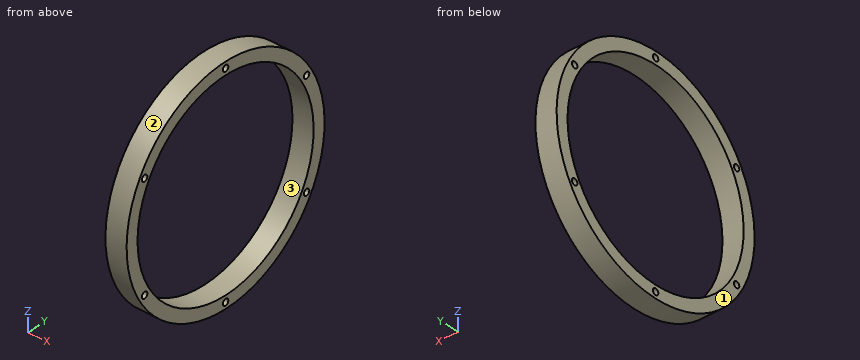
Autodesk Inventor part; units mm, degrees
ref_plane "YZ Plane" through (0, 0, 0) normal (1, 0, 0) x (0, 1, 0)
ref_plane "XZ Plane" through (0, 0, 0) normal (0, 1, 0) x (-1, 0, 0)
ref_plane "XY Plane" through (0, 0, 0) normal (0, 0, 1) x (1, 0, 0)
sketch "Sketch1" plane through (0, 0, 0) normal (0, 1, 0) x (-1, 0, 0)
  line L0 (0, -83.3) -> (0, -70.7) construction
  line L1 (-10.78, 0) -> (10.78, 0) construction
  line L2 (-7.7, -72.5) -> (7.7, -72.5)
  line L3 (-7.7, -72.5) -> (-7.7, -81.5)
  line L4 (-7.7, -81.5) -> (7.7, -81.5)
  line L5 (7.7, -81.5) -> (7.7, -72.5)
  dimension "d30" = 15.4
  dimension "d31" = 9
  dimension "d47" = 72.5
revolve "Revolution1" add sketch "Sketch1" angle 360 about axis through (0, 0, 0) along (-1, 0, 0)
sketch "Sketch2" plane through (-7.7, 0, 0) normal (-1, 0, 0) x (0, 0, 1)
  line L0 (0, 114.1) -> (0, -114.1) construction
  line L1 (-114.1, 0) -> (114.1, 0) construction
  circle A0 centre (0, 0) radius 72.5
  circle A1 centre (0, 0) radius 81.5
  circle A2 centre (0, 0) radius 77 construction
  point P0 (-77, 0)
  dimension "d33" = 4.5
  dimension "d34" = 4.5
hole "Hole1" at (-7.7, 0, -77) direction (1, 0, 0) diameter 4.5 end through all
pattern_circular "Circular Pattern1" count 6 over 360 about axis through (-10, 0, 0) along (1, 0, 0) of "Hole1"
equation "\"d33\" = d34"
equation "\"D_ring\" = D_ext"
properties part number "Adapter_stages_planetary" material "Aluminum 6061"
Input: part model. Units: mm. Frame: model coordinates. Face numbers are marked on the shaded views. Give positions to 0.01 mm unless a question says otherwise; leave off trailing zeros. Order: outer loops, then holes, each group sorted by start corner. A loop starts at its lowest first (then second) coordinate and runs counter-clockwise, first axis right, second up. Notation, with made-up numbers: (-37, 80) -> (-22, 80) arc R22 cw to (-22, 87) -> close; hole circle Ø4 at (-8, -27). An arc over 180 degrees is marked (long way). Use one line per item in the form item = value.
1) Line query: probe 1 along Z at (x, y) = (-6, 67); probe 2 along Z at (x, y) = (3.25, 37.5); probe 3 along Z at (x, y) = (4.5, -18). Output: solid intervals per line, ascending.
Response values:
probe_1 = -46.4 to -40.73, -36.27 to -27.7, 27.7 to 36.27, 40.73 to 46.4
probe_2 = -72.36 to -62.05, 62.05 to 72.36
probe_3 = -79.49 to -70.23, 70.23 to 79.49
2) Section D-D, the plane x = -1.75. Return loops of the section in (y, z) (3 decimals), and give its area (3 significant figures).
Response values:
outline = circle Ø163 at (0, 0); hole circle Ø145 at (0, 0); hole circle Ø4.5 at (-66.684, -38.5); hole circle Ø4.5 at (-66.684, 38.5); hole circle Ø4.5 at (0, -77); hole circle Ø4.5 at (0, 77); hole circle Ø4.5 at (66.684, -38.5); hole circle Ø4.5 at (66.684, 38.5)
area = 4,260 mm^2
3) First-contact query: pin 1 Ø6 at (x, z) = (3.5, 62) entering from -Y (3 decimals); pin 2 Ø4 at (x, y) = (3, -4) entering from +Z; pin 3 Ø6 at (x, z) = (-1.5, 42.5) entering from -Y. Flat tips, straight axial feed; report the tip coordinate or a pass-through.
Response values:
pin_1 = -56.225
pin_2 = 81.48
pin_3 = -71.29
4) Section A-A, the plane y = 0. Return loops of the section in (x, z).
Response values:
outline = (-7.7, -81.5) -> (7.7, -81.5) -> (7.7, -79.25) -> (-7.7, -79.25) -> close; (-7.7, -74.75) -> (7.7, -74.75) -> (7.7, -72.5) -> (-7.7, -72.5) -> close; (-7.7, 72.5) -> (7.7, 72.5) -> (7.7, 74.75) -> (-7.7, 74.75) -> close; (-7.7, 79.25) -> (7.7, 79.25) -> (7.7, 81.5) -> (-7.7, 81.5) -> close
5) Section C-C, the plane y = -22.5. Return loops of the section in (x, z).
Response values:
outline = (-7.7, -78.33) -> (7.7, -78.33) -> (7.7, -68.92) -> (-7.7, -68.92) -> close; (-7.7, 68.92) -> (7.7, 68.92) -> (7.7, 78.33) -> (-7.7, 78.33) -> close
6) Mould query, pull axis Z, two halves, no side actions, for the marked faces 1, 2 and 3. Classes: pulls with the +Z half, pulls with the -Z half, needs draft (parallel to the pull), parting line crosses it, or undercut.
Response values:
face_1 = needs draft
face_2 = parting line crosses it
face_3 = undercut
7) Section B-B, the plane z = 0. Return loops of the section in (x, y), and give its area (3 significant figures).
Response values:
outline = (-7.7, -81.5) -> (7.7, -81.5) -> (7.7, -72.5) -> (-7.7, -72.5) -> close; (-7.7, 72.5) -> (7.7, 72.5) -> (7.7, 81.5) -> (-7.7, 81.5) -> close
area = 277 mm^2
